The model under review builds one solid part; all positions refer to its coordinate system, in mm. A direction names the side the tool comes from. Coordinates: 2 decimals unless noted, no trailing zeros. Loops run counter-clockwise (first coordinate to the right, second up) from the corner with the lowest first, then second, coordinate; pieces in that order, holes last. Notation, with made-up numbers: (-19.5, -26) - (22.5, -26) arc R16 cw to (22.5, -1) - close; hole circle Ø8 at (-18.75, 67.5). An arc over 180 degrees is marked (long way). One line per item, written item: value. Start each with the question number.
1. We need section C-C, the plane y = 37. Give the boundary of the cut face in (x, z), then the cut area to 3 significant figures.
2. We need section D-D, the plane z = 87.5. Give the boundary of the cut face in (x, y).
3. Mouldability with a two-part tool opening along Z and no side actions: class faces 1 (the face through (-1, 134, 0)), 2 (the face through (-170, -2, 26)), 3 (the face through (-160.1, 85.4, 40.1)), 4 (the face through (-88.301, -141.619, 136.143)) as +Z half, -Z half, draft (parallel to the pull), parting line (faces both ways), or undercut.
4. For faces 5 (the face through (-70, 141, 113)), 6 (the face through (-104, -142, 129)), 7 (the face through (-160, 2, 66)), 8 (the face through (150, 2, 25)), list the 3-axis set-ups (+Z, -Z, +X, -X, +Y, -Y) from which the entire face can be reached by the end or side of a thin tool; tool diameter is ignored.
5. Insertion check: P1, Ø13.5, axis at x = -138.5, y = -138, coming from the +Z side; P2, Ø5, axis at y = -145, z = 134, coming from the +X side; P3, Ø8.5, axis at y = 141, z = 115, coming from the -X side. Each pin has a flat end and moves straight along its axis. Give the tip position at first contact, or say it passes through.
6. We need section A-A, the plane y = 80. Give the boundary of the cut face in (x, z), then the cut area to 3 significant figures.
7. To check wall thickness, follow line 1 (Y direction, x = -28.5, z = 43); line 2 (X direction, y = -12, z = 51). State the ranges of each line that lie inside material, in increasing order.
8. We need section B-B, the plane x = -87. Give the boundary of the cut face in (y, z), then the cut area to 3 significant figures.
Autodesk Inventor part; units mm, degrees
ref_plane "Work Plane1" through (-87, -150, 162) normal (0, 0, 1) x (1, 0, 0)
ref_plane "Work Plane2" through (-87, 133, 162) normal (0, 0, 1) x (1, 0, 0)
ref_plane "Work Plane3" through (-87, -150, 162) normal (0, 0, 1) x (1, 0, 0)
sketch "Sketch1" plane through (0, 0, 0) normal (0, 0, 1) x (1, 0, 0)
  line L0 (150, -133) -> (-150, -133)
  line L1 (-150, -133) -> (-150, 133)
  line L2 (-150, 133) -> (150, 133)
  line L3 (150, 133) -> (150, -133)
  line L4 (0, 0) -> (0, 56.2774)
  line L5 (0, 0) -> (78.3407, 0)
  line L6 (170, -150) -> (-170, -150)
  line L7 (-170, -150) -> (-170, 150)
  line L8 (-170, 150) -> (170, 150)
  line L9 (170, 150) -> (170, -150)
  point P0 (0, 133)
  point P1 (150, 0)
  dimension "d0" = 300
  dimension "d1" = 266
  dimension "d2" = 17
  dimension "d3" = 17
  dimension "d4" = 20
  dimension "d5" = 20
extrude "Extrusion1" add sketch "Sketch1" along normal blind 66
sketch "Sketch2" plane through (-170, -150, 0) normal (-1, 0, 0) x (0, 0, 1)
  circle A0 centre (46, 230) radius 8
  circle A1 centre (46, 70) radius 8
  circle A2 centre (46, 230) radius 8
  circle A3 centre (46, 70) radius 8
  circle A4 centre (40, 150) radius 9.5
  circle A5 centre (40, 150) radius 9.5
  point P0 (0, 150)
extrude "Extrusion2" cut sketch "Sketch2" against normal through all
sketch "Sketch4" plane through (0, 0, 66) normal (0, 0, 1) x (1, 0, 0)
  line L0 (150, -133) -> (-150, -133)
  line L1 (170, 150) -> (-170, 150)
  line L2 (-170, 150) -> (-170, -150)
  line L3 (-70, -150) -> (-170, -150)
  line L4 (-170, -150) -> (-170, -133)
  line L5 (-170, -133) -> (-70, -133)
  line L6 (-70, -133) -> (-70, -150)
  line L7 (-70, 133) -> (-170, 133)
  line L8 (-170, 133) -> (-170, 150)
  line L9 (-170, 150) -> (-70, 150)
  line L10 (-70, 150) -> (-70, 133)
  point P0 (0, 0)
  dimension "d14" = 100
  dimension "d15" = 17
  dimension "d17" = 100
  dimension "d18" = 17
extrude "Extrusion3" add sketch "Sketch4" along normal blind 30
ref_plane "Work Plane1" through (-87, -150, 162) normal (0, 0, 1) x (1, 0, 0)
ref_plane "Work Plane2" through (-87, 133, 162) normal (0, 0, 1) x (1, 0, 0)
ref_plane "Work Plane3" through (-87, -150, 162) normal (0, 0, 1) x (1, 0, 0)
sketch "Sketch9" plane through (0, 0, 96) normal (0, 0, 1) x (1, 0, 0)
  line L0 (-70, 133) -> (-70, 150)
  line L1 (-70, 150) -> (-170, 150)
  line L2 (-104, 133) -> (-104, 150)
  line L3 (-70, 133) -> (-104, 133)
  line L4 (-104, 133) -> (-104, 150)
  line L5 (-104, 150) -> (-70, 150)
  line L6 (-70, 150) -> (-70, 133)
  point P0 (0, 0)
ref_plane "Work Plane4" through (-157, 133, 162) normal (0, 0, 1) x (1, 0, 0)
extrude "Extrusion8" add sketch "Sketch9" along normal up to surface (66 mm away)
sketch "Sketch10" plane through (0, 0, 96) normal (0, 0, 1) x (1, 0, 0)
  line L0 (-70, -150) -> (-70, -133)
  line L1 (-70, -133) -> (-170, -133)
  line L2 (-104, -150) -> (-104, -133)
  line L3 (-70, -150) -> (-104, -150)
  line L4 (-104, -150) -> (-104, -133)
  line L5 (-104, -133) -> (-70, -133)
  line L6 (-70, -133) -> (-70, -150)
  point P0 (0, 0)
ref_plane "Work Plane5" through (-157, -150, 162) normal (0, 0, 1) x (1, 0, 0)
extrude "Extrusion9" add sketch "Sketch10" along normal up to surface (66 mm away)
sketch "Sketch11" plane through (-170, -150, 0) normal (0, -1, 0) x (1, 0, 0)
  circle A0 centre (83, 142) radius 6
  point P0 (170, 0)
extrude "Extrusion10" cut sketch "Sketch11" against normal through all
sketch "Sketch12" plane through (0, 0, 0) normal (0, 1, 0) x (-1, 0, 0)
  point P0 (0, 0)
properties part number "Base" material "Wood (Birch)"
Findings below:
1. outline: (-170, 0) - (-150, 0) - (-150, 66) - (-170, 66) - close; (150, 0) - (170, 0) - (170, 66) - (150, 66) - close
1. area: 2,640 mm2
2. outline: (-170, -150) - (-70, -150) - (-70, -133) - (-170, -133) - close; (-170, 133) - (-70, 133) - (-70, 150) - (-170, 150) - close
3. face 1: -Z half
3. face 2: draft
3. face 3: undercut
3. face 4: undercut
4. face 5: +Z, +X, +Y, -Y
4. face 6: +Z, -X, +Y, -Y
4. face 7: +Z, +X, -X
4. face 8: +Z, -Z
5. P1: z = 96
5. P2: x = -70
5. P3: x = -104
6. outline: (-170, 0) - (-150, 0) - (-150, 38) - (-170, 38) - close; (-170, 54) - (-150, 54) - (-150, 66) - (-170, 66) - close; (150, 0) - (170, 0) - (170, 38) - (150, 38) - close; (150, 54) - (170, 54) - (170, 66) - (150, 66) - close
6. area: 2,000 mm2
7. line 1: -150 to -133, 133 to 150
7. line 2: -170 to -150, 150 to 170
8. outline: (-150, 0) - (-133, 0) - (-133, 136) - (-150, 136) - close; (-150, 148) - (-133, 148) - (-133, 162) - (-150, 162) - close; (133, 0) - (150, 0) - (150, 136) - (133, 136) - close; (133, 148) - (150, 148) - (150, 162) - (133, 162) - close
8. area: 5,100 mm2
